Check sheet for the drawn part. Datum: minimum x, y, z corner. Units: mm. A direction names the side the tool comes from. Coordinates: 2 decimals unless noted, no trailing zeros. Loops run counter-clockwise (first coordinate to the right, second up) from the corner with the lowest first, then second, coordinate; pieces in that order, holes last. Notation, with made-up numbers: (86.5, 58.5) - (128.5, 58.5) arc R20 ccw to (128.5, 74.5) - close; hole circle Ø5 at (72.5, 52.25). An arc over 180 degrees is marked (long way). Answer as CSV lines item,"result". Start each with the question number.
1. Cross-section at D-D (z = 17.75). Enter the section's corners in (x, y), plus the area to 3 significant figures.
2. Cross-section at A-A (z = 3). Enter the section's corners in (x, y), plus the area to 3 significant figures.
3. Set-up check for the marked faces 1, 2 and 3: record each of +Z, -Z, +X, -X, +Y, -Y from which the full face is reachable in a straight line by a thin tool's end or side.
4. Cross-section at B-B (x = 44). Enter the section's corners in (y, z), plus the area to 3 significant figures.
5. Cross-section at C-C (y = 34.5). Enter the section's corners in (x, z).
6. Gauge pin test, flat ends, axial feed: P1, Ø6, axis at x = 47, y = 14.5, coming from the -Z side; P2, Ø4, axis at y = 9.5, z = 2, coming from the +X side; P3, Ø4, axis at y = 29.5, z = 19, coming from the +X side; P4, Ø1.5, axis at x = 14, z = 13.5, coming from the +Y side. Record the tip position at first contact, or that the pin passes through.
7. Material ranges on line 1 (Z direction, x = 90.5, y = 61.5); line 2 (X direction, y = 41.5, z = 22.25); line 3 (Z direction, x = 19.5, y = 47), recorded low to high. Write a range as [from, to].
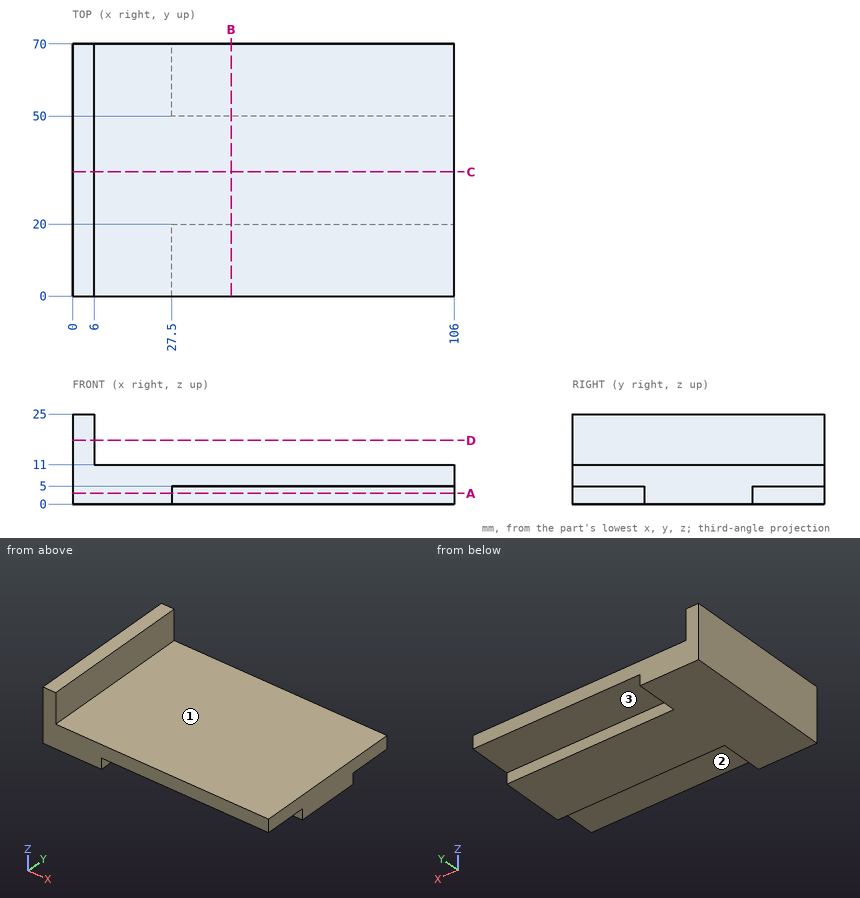
Values follow:
1,outline,"(0, 0) - (6, 0) - (6, 70) - (0, 70) - close"
1,area,"420 mm²"
2,outline,"(0, 0) - (27.5, 0) - (27.5, 20) - (106, 20) - (106, 50) - (27.5, 50) - (27.5, 70) - (0, 70) - close"
2,area,"4,280 mm²"
3,face 1,"+Z, +X, +Y, -Y"
3,face 2,"-Z, +X, -Y"
3,face 3,"-Z, +X, +Y"
4,outline,"(0, 5) - (20, 5) - (20, 0) - (50, 0) - (50, 5) - (70, 5) - (70, 11) - (0, 11) - close"
4,area,"570 mm²"
5,outline,"(0, 0) - (106, 0) - (106, 11) - (6, 11) - (6, 25) - (0, 25) - close"
6,P1,"stops at z = 5"
6,P2,"stops at x = 27.5"
6,P3,"stops at x = 6"
6,P4,"passes through"
7,line 1,"z = [5, 11]"
7,line 2,"x = [0, 6]"
7,line 3,"z = [0, 11]"
